```python
from build123d import *

# Parameters (mm, degrees)
F1_DEPTH       = 50.8
F3_D           = 6.096
F3_CBORE_D     = 12.7
F3_CBORE_DEPTH = 7.9248
F5_DEPTH       = 132.571551198
F7_DEPTH       = 53.1231379703


with BuildPart() as f1:
    # F0 (on Front) → F1 (new body)
    with BuildSketch(Plane.XZ):
        Polygon((0, 12.7), (0, 0), (85.852, 0), (130.3175357378, -44.4655357378), (148.2780479799, -26.5050234956), (116.9623968646, 3.8574382814), (108.1219795526, -5.2605122421), (90.1614673105, 12.7), align=None)
    extrude(amount=F1_DEPTH)

    # F3 (through all)
    with Locations(Plane(origin=(0, 0, 0), x_dir=(1, 0, 0), z_dir=(0, 0, -1))):
        with Locations((15.748, 38.1), (15.748, 12.7), (69.596, 12.7), (69.596, 38.1)):
            CounterBoreHole(F3_D / 2, F3_CBORE_D / 2, F3_CBORE_DEPTH)

    # F4 (on face) → F5 (cut, through all)
    with BuildSketch(Plane(origin=(87.3915357378, 0, -87.3915357378), x_dir=(0, 1, 0), z_dir=(0.7071067812, 0, -0.7071067812))):
        Polygon((-15.748, 86.1065313784), (-35.052, 86.1065313784), (-35.052, 80.0105313784), (-41.148, 80.0105313784), (-41.148, 73.4065313784), (-25.4, 73.4065313784), (-9.652, 73.4065313784), (-9.652, 80.0105313784), (-15.748, 80.0105313784), align=None)
    extrude(amount=-F5_DEPTH, mode=Mode.SUBTRACT)

    # F6 (on face) → F7 (cut, through all)
    with BuildSketch(Plane(origin=(42.926, 0, 42.926), x_dir=(0, -1, 0), z_dir=(-0.7071067812, 0, -0.7071067812))):
        with BuildLine():
            ThreePointArc((25.4, -123.590295077), (12.3070777205, -121.9743014541), (0, -117.2233134317))
            Line((0, -117.2233134317), (0, -123.590295077))
            Line((0, -123.590295077), (25.4, -123.590295077))
        make_face()
        with BuildLine():
            ThreePointArc((50.8, -117.2233134317), (38.4929222795, -121.9743014541), (25.4, -123.590295077))
            Line((25.4, -123.590295077), (50.8, -123.590295077))
            Line((50.8, -123.590295077), (50.8, -117.2233134317))
        make_face()
    extrude(amount=-F7_DEPTH, mode=Mode.SUBTRACT)


solid = f1.part
```
For this review, take the finished solid that the model builds, in its own axes (mm). A direction names the side the tool comes from. Coordinates: 2 decimals unless noted, no trailing zeros. Loops run counter-clockwise (first coordinate to the right, second up) from the corner with the lowest first, then second, coordinate; pieces in that order, holes last.
1. Add section C-C, the plane z = -17. Give the boundary of the cut face in (x, y), then the cut area to 3 significant figures.
2. For faces 4 (the flat face through (42, -25, 0)), 5 (the flat face through (131, -15.748, -13)), 6 (the flat face through (126, -41.148, -17)), 7 (the cylindrical face through (18.678, -32.466, 3.907)), list the 3-axis set-ups (+Z, -Z, +X, -X, +Y, -Y) from which the entire face can be reached by the end or side of a thin tool; tool diameter is ignored.
3. Add section A-A, the plane x = 70.5. Give the boundary of the cut face in (y, z).
4. For line 1 (Y direction, x = 124, z = -4); line 2 (X direction, y = -38.1, z = 10.5); line 3 (X direction, y = -38.1, z = 5.75), list the stretches that pass through material, from the lowest coordinate up.
5. Add section D-D, the plane y = -43. Give the boundary of the cut face in (x, z).
6. Add section B-B, the plane y = -12.7. Give the boundary of the cut face in (x, z), then the cut area to 3 significant figures.
7. Mouldability with a two-part tool opening along X and no side actions: class faces 1 (the flat face through (99.27, -25.04, 3.59)), 2 (the flat face through (0, -25, 6)), 3 (the flat face through (46, -25, 12.7)) as +X half, -X half, draft (parallel to the pull), parting line (faces both ways), or undercut.
8. Insertion check: P1, Ø10, axis at x = 66.5, y = -39.5, coming from the -Z side; P2, Ø5, axis at y = -28, z = -24, coming from the -X side; P3, Ø11.5, axis at x = 15.748, y = -38.1, coming from the +Z side; P4, Ø8, axis at x = 15.748, y = -38.1, coming from the -Z side. Each pin has a flat end and moves straight along its axis. Give the tip position at first contact, or say it passes through.
Result:
1. outline: (102.85, -50.8) - (138.47, -50.8) - (138.47, -35.05) - (130.15, -35.05) - (130.15, -41.15) - (120.81, -41.15) - (120.81, -9.65) - (130.15, -9.65) - (130.15, -15.75) - (138.47, -15.75) - (138.47, 0) - (102.85, 0) - close
1. area: 1,350 mm2
2. face 4: -Z, -X, +Y, -Y
2. face 5: +Z, +X
2. face 6: none
2. face 7: -Z
3. outline: (-50.8, 0) - (-44.39, 0) - (-44.39, 7.92) - (-41.01, 7.92) - (-41.01, 12.7) - (-50.8, 12.7) - close; (-35.19, 7.92) - (-31.81, 7.92) - (-31.81, 0) - (-18.99, 0) - (-18.99, 7.92) - (-15.61, 7.92) - (-15.61, 12.7) - (-35.19, 12.7) - close; (-9.79, 7.92) - (-6.41, 7.92) - (-6.41, 0) - (0, 0) - (0, 12.7) - (-9.79, 12.7) - close
4. line 1: y = -50.8 to -35.05, -15.75 to 0
4. line 2: x = 0 to 12.7, 18.8 to 66.55, 72.64 to 92.36
4. line 3: x = 0 to 9.4, 22.1 to 63.25, 75.95 to 97.11
5. outline: (0, 0) - (11.71, 0) - (11.71, 7.92) - (19.79, 7.92) - (19.79, 0) - (65.56, 0) - (65.56, 7.92) - (73.63, 7.92) - (73.63, 0) - (85.85, 0) - (128.23, -42.37) - (146.15, -24.45) - (116.96, 3.86) - (108.12, -5.26) - (90.16, 12.7) - (0, 12.7) - close
6. outline: (0, 0) - (9.4, 0) - (9.4, 7.92) - (12.7, 7.92) - (12.7, 12.7) - (0, 12.7) - close; (18.8, 7.92) - (22.1, 7.92) - (22.1, 0) - (63.25, 0) - (63.25, 7.92) - (66.55, 7.92) - (66.55, 12.7) - (18.8, 12.7) - close; (72.64, 7.92) - (75.95, 7.92) - (75.95, 0) - (85.85, 0) - (129.24, -43.39) - (138.22, -34.41) - (108.59, -4.78) - (108.12, -5.26) - (90.16, 12.7) - (72.64, 12.7) - close; (113.19, -0.04) - (142.89, -29.74) - (147.19, -25.45) - (116.96, 3.86) - close
6. area: 1,900 mm2
7. face 1: undercut
7. face 2: -X half
7. face 3: draft
8. P1: stops at z = 0
8. P2: stops at x = 107.35
8. P3: stops at z = 12.7
8. P4: stops at z = 7.92
